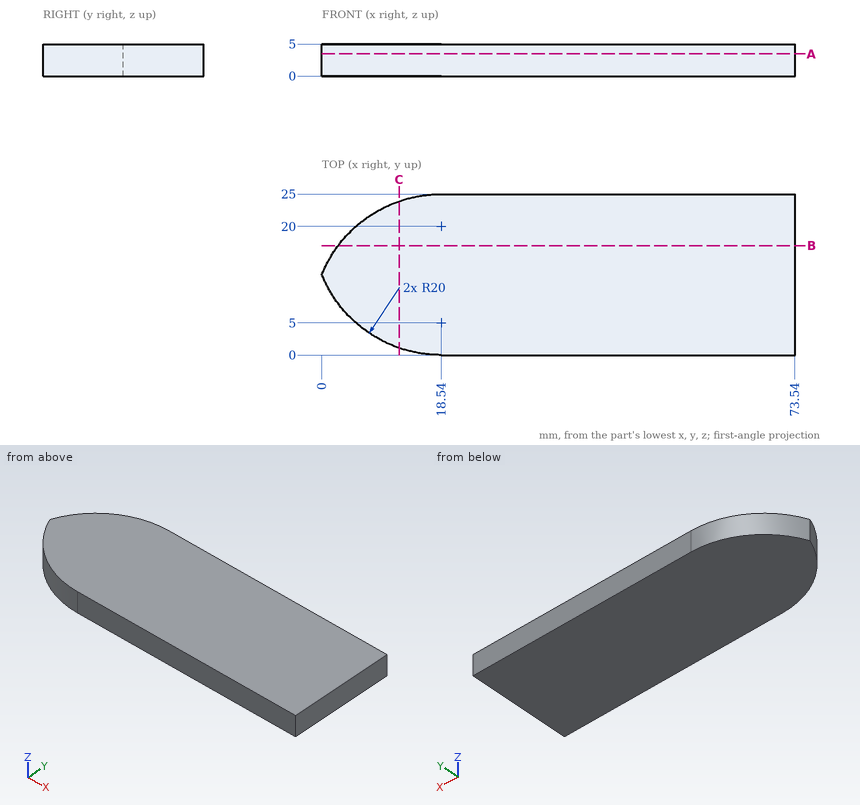
Print and shaded views of the part. All mm, measured from the part's lowest x, y and z. Coordinates: 2 decimals unless noted, no trailing zeros. Order: outer loops, then holes, each group sorted by start corner. A loop starts at its lowest first (then second) coordinate and runs counter-clockwise, first axis right, second up. Notation, with made-up numbers: M -4.5,56.25 L 47.5,56.25 A28 ccw 47.5,81.25 Z; hole C 56,-24.5 d8. An arc over 180 degrees is marked long. Answer as CSV lines item,"result".
1) Cut at A-A (z = 3.45). List the corners of the cut face in (x, y), then the cut area to 3 significant figures.
Verdict:
outline,"M 0,12.5 A20 ccw 18.54,0 L 73.54,0 L 73.54,25 L 18.54,25 A20 ccw Z"
area,"1,710 mm2"
2) Cut at C-C (x = 12). List the corners of the cut face in (y, z), then the cut area to 3 significant figures.
Verdict:
outline,"M 1.1,0 L 23.9,0 L 23.9,5 L 1.1,5 Z"
area,"114 mm2"
3) Flat gauge pin, fed straight in: P1, Ø1, axis at x = 33.5, y = 3.5, coming from the -Z side. Where does the tip first touch, or does it go through?
Verdict:
P1,"z = 0"
4) Drill centre lines: L1, parallel to Y at x = 11.5, z = 4.6; L2, parallel to X at y = 5.5, z = 0.6 (1 decimal); L3, parallel to X at y = 19.25, z = 1.15 (1 decimal). Where is each one in solid material? Low to high. Write a range as from..to.
Verdict:
L1,"1.28..23.72"
L2,"4.8..73.5"
L3,"4.5..73.5"
5) Cut at B-B (y = 17). List the corners of the cut face in (x, z), then the cut area to 3 significant figures.
Verdict:
outline,"M 2.54,0 L 73.54,0 L 73.54,5 L 2.54,5 Z"
area,"355 mm2"
